from build123d import *

# Parameters (mm, degrees)
FRAME_EXTERIOR_MASTER_OUTLINE_R = 19.685
FRAME_EXTERIOR_MASTER_DEPTH     = 6.35
CUT_EXTRUDE1_DEPTH              = 611.690430988


# Read off the part's stored shape, not the designer's step: Frame Exterior Master
with BuildPart() as part:
    # Frame Exterior Master outline → Frame Exterior Master (new body)
    with BuildSketch(Plane.XY):
        Polygon((431.8, 12.7), (431.8, 431.8), (215.9, 431.8), (0, 304.8), (0, 12.7), (127, 12.7), (127, 50.8), (254, 50.8), (254, 12.7), align=None)
        with Locations((98.15, 150.3)):
            Circle(FRAME_EXTERIOR_MASTER_OUTLINE_R, mode=Mode.SUBTRACT)
        with Locations((333.65, 150.3)):
            Circle(FRAME_EXTERIOR_MASTER_OUTLINE_R, mode=Mode.SUBTRACT)
    extrude(amount=FRAME_EXTERIOR_MASTER_DEPTH)

    # Sketch1 → Cut-Extrude1 (cut, through all)
    with BuildSketch(Plane(origin=(0, 0, 0), x_dir=(-1, 0, 0), z_dir=(0, 0, -1))):
        Polygon((-406.4, 406.4), (-406.4, 190.5), (-25.4, 190.5), (-25.4, 290.27257022), (-222.816630625, 406.4), align=None)
    extrude(amount=-CUT_EXTRUDE1_DEPTH, mode=Mode.SUBTRACT)


solid = part.part
Here's how the part is built. I have some questions about the finished solid (model axes, mm). Give positions to 0.01 mm unless a question says otherwise; leave off trailing zeros. Loops run counter-clockwise (first coordinate to the right, second up) from the corner with the lowest first, then second, coordinate; pieces in that order, holes last. Notation, with made-up numbers: (-9, 35) -> (18, 35) arc R21 ccw to (18, 43) -> close; hole circle Ø10 at (-22.5, -9). An arc over 180 degrees is marked (long way). One line per item, written item: value.
Q1. We'd pull the mould along X, two halves only. Please class faces 1 (the face through (109.46, 369.19, 3.13)), 2 (the face through (213, 179, 6.35)), 3 (the face through (122.726, 347.523, 3.131)): pulls with the +X half, pulls with the -X half, needs draft (parallel to the pull), parting line crosses it, or undercut.
Answers follow:
face 1: pulls with the -X half
face 2: needs draft
face 3: undercut
Q2. Suppose I cut it at D-D on y = 233. Please give me the cut outline in (x, z).
Answers follow:
outline: (0, 0) -> (25.4, 0) -> (25.4, 6.35) -> (0, 6.35) -> close; (406.4, 0) -> (431.8, 0) -> (431.8, 6.35) -> (406.4, 6.35) -> close
Q3. I'm going to push flat-ended pins straight in: pin 1 Ø1.5 at (y, z) = (339, 1) entering from -X (3 decimals); pin 2 Ø1 at (y, z) = (355, 3.5) entering from -X. Where does each tip first touch, or does it pass through?
Answers follow:
pin 1: x = 56.865
pin 2: x = 84.49
Q4. Suppose I cut it at B-B on y = 150.3. Please give me the cut outline in (x, z) (3 decimals).
Answers follow:
outline: (0, 0) -> (78.465, 0) -> (78.465, 6.35) -> (0, 6.35) -> close; (117.835, 0) -> (313.965, 0) -> (313.965, 6.35) -> (117.835, 6.35) -> close; (353.335, 0) -> (431.8, 0) -> (431.8, 6.35) -> (353.335, 6.35) -> close
Q5. Suppose I cut it at A-A on x = 333.65. Please give me the cut outline in (y, z) (3 decimals), then the cut area to 3 significant figures.
Answers follow:
outline: (12.7, 0) -> (130.615, 0) -> (130.615, 6.35) -> (12.7, 6.35) -> close; (169.985, 0) -> (190.5, 0) -> (190.5, 6.35) -> (169.985, 6.35) -> close; (406.4, 0) -> (431.8, 0) -> (431.8, 6.35) -> (406.4, 6.35) -> close
area: 1,040 mm^2
Q6. If I drill on line 1 along Y through (x, z) = (333.65, 4.5) (3 decimals); line 2 along Y through (x, z) = (91, 5); line 3 along X through (y, z) = (260.5, 4.75), over which ranges is the centre line in solid material (lowest first)?
Answers follow:
line 1: 12.7 to 130.615, 169.985 to 190.5, 406.4 to 431.8
line 2: 12.7 to 131.96, 168.64 to 190.5, 328.86 to 358.33
line 3: 0 to 25.4, 406.4 to 431.8
Q7. Suppose I cut it at C-C on z = 3.5. Please give me the cut outline in (x, y) (3 decimals), then the cut area to 3 significant figures.
Answers follow:
outline: (0, 12.7) -> (127, 12.7) -> (127, 50.8) -> (254, 50.8) -> (254, 12.7) -> (431.8, 12.7) -> (431.8, 431.8) -> (215.9, 431.8) -> (0, 304.8) -> close; hole (25.4, 190.5) -> (406.4, 190.5) -> (406.4, 406.4) -> (222.817, 406.4) -> (25.4, 290.273) -> close; hole circle Ø39.37 at (98.15, 150.3); hole circle Ø39.37 at (333.65, 150.3)
area: 89,200 mm^2
